Here's how the part is built. I have some questions about the finished solid (model axes, mm). Round coordinates to 2 decimals unless told otherwise and drop trailing zeros. Order: outer loops, then holes, each group sorted by start corner. A loop starts at its lowest first (then second) coordinate and runs counter-clockwise, first axis right, second up.
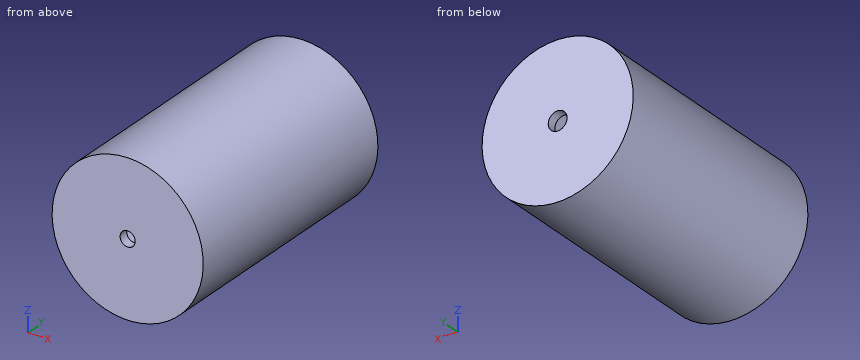
```python
from build123d import *

# Parameters (mm, degrees)
SKETCH1_R           = 8
BOSS_EXTRUDE1_DEPTH = 26.4
SHELL7_T            = 1
SKETCH4_R           = 1
CUT_EXTRUDE1_DEPTH  = 3
SKETCH6_R           = 0.8
CUT_EXTRUDE2_DEPTH  = 6


with BuildPart() as part:
    # Sketch1 → Boss-Extrude1 (new body)
    with BuildSketch(Plane(origin=(0, 0, 0), x_dir=(1, 0, 0), z_dir=(0, 1, 0))):
        with Locations(Location((0, 0, 0), (0, 0, 270))):
            Circle(SKETCH1_R)
    extrude(amount=BOSS_EXTRUDE1_DEPTH)

    # Shell7 (no face opened: a closed hollow body)
    add(offset(amount=-SHELL7_T, mode=Mode.PRIVATE), mode=Mode.SUBTRACT)

    # Sketch4 → Cut-Extrude1 (cut)
    with BuildSketch(Plane(origin=(0, 26.4, 0), x_dir=(1, 0, 0), z_dir=(0, 1, 0))):
        with Locations(Location((0, 0, 0), (0, 0, 270))):
            Circle(SKETCH4_R)
    extrude(amount=-CUT_EXTRUDE1_DEPTH, mode=Mode.SUBTRACT)

    # Sketch6 → Cut-Extrude2 (cut)
    with BuildSketch(Plane.XZ):
        with Locations(Location((0, 0, 0), (0, 0, 270))):
            Circle(SKETCH6_R)
    extrude(amount=-CUT_EXTRUDE2_DEPTH, mode=Mode.SUBTRACT)


solid = part.part
```
1. I'm going to push flat-ended pins straight in: P1, Ø1.5, axis at y = 8, z = 2.5, coming from the -X side; P2, Ø6, axis at x = -4.5, y = 3, coming from the +Z side; P3, Ø5, axis at x = 3.5, y = 17.5, coming from the -Z side. Where does each tip first touch, or does it pass through?
Evaluation:
P1: stops at x = -7.81
P2: stops at z = 7.86
P3: stops at z = -7.94
2. If we section it at B-B, the plane z = 0: Write out the boundary of the cut face in (x, y).
Evaluation:
outline: (-8, 0) - (-0.8, 0) - (-0.8, 1) - (-7, 1) - (-7, 25.4) - (-1, 25.4) - (-1, 26.4) - (-8, 26.4) - close; (0.8, 0) - (8, 0) - (8, 26.4) - (1, 26.4) - (1, 25.4) - (7, 25.4) - (7, 1) - (0.8, 1) - close
3. If we section it at D-D, the plane x = -3.75: Write out the boundary of the cut face in (y, z).
Evaluation:
outline: (0, -7.07) - (26.4, -7.07) - (26.4, 7.07) - (0, 7.07) - close; hole (1, -5.91) - (25.4, -5.91) - (25.4, 5.91) - (1, 5.91) - close
4. If we section it at C-C, the plane y = 6: Write out the boundary of the cut face in (x, z), and give its area (3 significant figures).
Evaluation:
outline: circle Ø16 at (0, 0); hole circle Ø14 at (0, 0)
area: 47.1 mm2
5. If we section it at A-A, the plane x = 0: Write out the boundary of the cut face in (y, z).
Evaluation:
outline: (0, -8) - (26.4, -8) - (26.4, -1) - (25.4, -1) - (25.4, -7) - (1, -7) - (1, -0.8) - (0, -0.8) - close; (0, 0.8) - (1, 0.8) - (1, 7) - (25.4, 7) - (25.4, 1) - (26.4, 1) - (26.4, 8) - (0, 8) - close
6. I need wall thicknesses on probe 1 along Y at (x, z) = (5, 1.25); probe 2 along X at (y, z) = (18.5, 0); probe 3 along X at (y, z) = (0.6, 0). Which ranges of each line are inside material? Lowest first, please.
Evaluation:
probe 1: y = 0 to 1, 25.4 to 26.4
probe 2: x = -8 to -7, 7 to 8
probe 3: x = -8 to -0.8, 0.8 to 8
